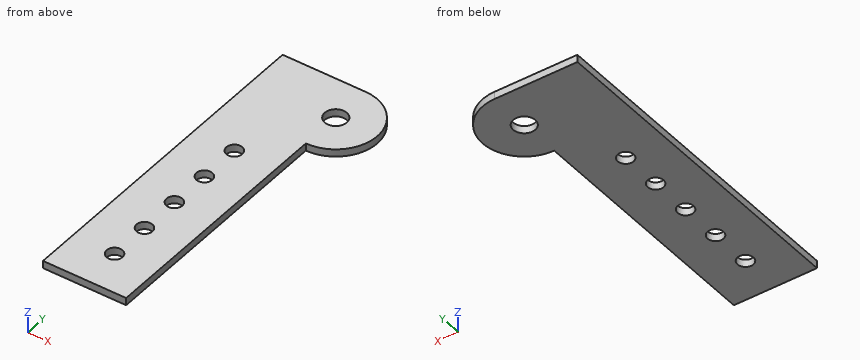
Autodesk Inventor part; units mm, degrees
ref_plane "YZ Plane" through (0, 0, 0) normal (1, 0, 0) x (0, 1, 0)
ref_plane "XZ Plane" through (0, 0, 0) normal (0, 1, 0) x (-1, 0, 0)
ref_plane "XY Plane" through (0, 0, 0) normal (0, 0, 1) x (1, 0, 0)
sketch "Sketch1" plane through (0, 0, 0) normal (0, 0, 1) x (1, 0, 0)
  line L0 (0, 0) -> (25.4, 0)
  line L1 (25.4, 0) -> (25.4, 101.6)
  line L2 (25.4, 101.6) -> (0, 101.6)
  line L3 (0, 101.6) -> (0, 0)
  arc A0 (25.4, 76.2) -> (25.4, 101.6) centre (25.4, 88.9) ccw
  dimension "d0" = 101.6
  dimension "d1" = 25.4
  dimension "d2" = 25.4
extrude "Extrusion1" add sketch "Sketch1" along normal blind 2.286
sketch "Sketch3" plane through (0, 0, 2.286) normal (0, 0, 1) x (1, 0, 0)
  line L0 (0, 101.6) -> (0, 0)
  line L1 (0, 0) -> (25.4, 0)
  line L2 (25.4, 101.6) -> (0, 101.6)
  point P0 (12.7, 63.5)
  point P1 (12.7, 50.8)
  point P2 (12.7, 38.1)
  point P3 (12.7, 25.4)
  point P4 (12.7, 12.7)
  dimension "d39" = 38.1
  dimension "d40" = 12.7
  dimension "d43" = 12.7
hole "Hole1" at (12.7, 63.5, 2.286) at (12.7, 50.8, 2.286) at (12.7, 38.1, 2.286) at (12.7, 25.4, 2.286) at (12.7, 12.7, 2.286) direction (0, 0, -1) diameter 4.8514 end through all
sketch "Sketch4" plane through (0, 0, 2.286) normal (0, 0, 1) x (1, 0, 0)
  line L0 (25.4, 0) -> (25.4, 76.2)
  arc A0 (25.4, 76.2) -> (25.4, 101.6) centre (25.4, 88.9) ccw
  point P0 (0, 0)
hole "Hole2" at (25.4, 88.9, 2.286) direction (0, 0, -1) diameter 6.7564 end through all
equation "\"d2\" = d1"
properties part number "Lifter Bracket" material "Aluminum 6061"
Read the model definition and answer for the solid it produces. Units are mm, in the model's axes. Round coordinates to 2 decimals unless told otherwise and drop trailing zeros. Write each loop counter-clockwise with the first axis right and the second up, starting at its lowest first coordinate (ties: lowest second). Pieces come first, ordered by that corner, then holes.
1. The part is cut by section B-B, the plane z = 1.7. Determine the outline of the cut face in (x, y), then the cut area to 3 significant figures.
2. Given pin 1 Ø4 at (x, y) = (12.7, 38.1) entering from +Z, flat-ended and moving along its own axis, determine where the tip first touches the part or whether it passes through.
3. Straight lines are drawn through the part: L1, parallel to Y at x = 12.7, z = 1.8; L2, parallel to X at y = 25.4, z = 0.75; L3, parallel to Y at x = 25.5, z = 1.4. For each, find the intervals that lie inside material, in ascending order.
4. The part is cut by section C-C, the plane y = 32.5. Determine the outline of the cut face in (x, z).
5. The part is cut by section D-D, the plane y = 50.5. Determine the outline of the cut face in (x, z).
6. The part is cut by section A-A, the plane y = 63.5. Determine the outline of the cut face in (x, z), then the cut area to 3 significant figures.
Values:
1. outline: (0, 0) - (25.4, 0) - (25.4, 76.2) arc R12.7 ccw to (25.4, 101.6) - (0, 101.6) - close; hole circle Ø4.85 at (12.7, 12.7); hole circle Ø4.85 at (12.7, 25.4); hole circle Ø4.85 at (12.7, 38.1); hole circle Ø4.85 at (12.7, 50.8); hole circle Ø4.85 at (12.7, 63.5); hole circle Ø6.76 at (25.4, 88.9)
1. area: 2,710 mm2
2. pin 1: passes through
3. L1: y = 0 to 10.27, 15.13 to 22.97, 27.83 to 35.67, 40.53 to 48.37, 53.23 to 61.07, 65.93 to 101.6
3. L2: x = 0 to 10.27, 15.13 to 25.4
3. L3: y = 76.2 to 85.52, 92.28 to 101.6
4. outline: (0, 0) - (25.4, 0) - (25.4, 2.29) - (0, 2.29) - close
5. outline: (0, 0) - (10.29, 0) - (10.29, 2.29) - (0, 2.29) - close; (15.11, 0) - (25.4, 0) - (25.4, 2.29) - (15.11, 2.29) - close
6. outline: (0, 0) - (10.27, 0) - (10.27, 2.29) - (0, 2.29) - close; (15.13, 0) - (25.4, 0) - (25.4, 2.29) - (15.13, 2.29) - close
6. area: 47.0 mm2
